```python
from build123d import *

# Parameters (mm, degrees)
EXTRUDE_1_DEPTH = 750


with BuildPart() as part:
    # Эскиз1 → Бобышка-Вытянуть1 (new body)
    with BuildSketch(Plane.XY):
        with BuildLine():
            Line((10, 14.5), (10, 13.5))
            ThreePointArc((10, 13.5), (9.853553391, 13.146446609), (9.5, 13))
            Line((9.5, 13), (-12.5, 13))
            ThreePointArc((-12.5, 13), (-12.853553391, 12.853553391), (-13, 12.5))
            Line((-13, 12.5), (-13, -9.5))
            ThreePointArc((-13, -9.5), (-13.146446609, -9.853553391), (-13.5, -10))
            Line((-13.5, -10), (-14.5, -10))
            ThreePointArc((-14.5, -10), (-14.853553391, -9.853553391), (-15, -9.5))
            Line((-15, -9.5), (-15, 15))
            Line((-15, 15), (9.5, 15))
            ThreePointArc((9.5, 15), (9.853553391, 14.853553391), (10, 14.5))
        make_face()
    extrude(amount=EXTRUDE_1_DEPTH)


solid = part.part
```
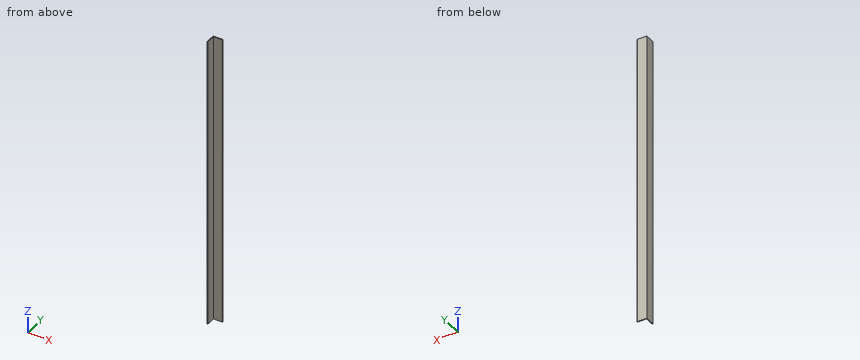
Can you work these out from the model? Positions are in its coordinate system, mm. Round coordinates to 2 decimals unless told otherwise and drop trailing zeros. Order: outer loops, then holes, each group sorted by start corner. A loop starts at its lowest first (then second) coordinate and runs counter-clockwise, first axis right, second up. Notation, with made-up numbers: (-35, -23.75) -> (6, -23.75) arc R28 cw to (6, 10.25) -> close; hole circle Ø1 at (69, 71). An arc over 180 degrees is marked (long way). Return JSON: item names as keys, results as strings. Group by question number.
1. If we section it at B-B, the plane y = -2.25: Write out the boundary of the cut face in (x, z), then the cut area to 3 significant figures.
2. If we section it at A-A, the plane z = 658.5: Write out the boundary of the cut face in (x, y).
3. If we section it at C-C, the plane x = -0.5: Write out the boundary of the cut face in (y, z), then the cut area to 3 significant figures.
4. Will this pin go through, and if not, where does the flat tip stop? pin 1 (3 mm diameter, centred on x = 7.5, z = 254, fed in from -Y).
5. I need wall thicknesses on line 1 (X direction, y = -5.5, z = 644); line 2 (Y direction, x = -0.75, z = 127). Which ranges of each line are inside material? Lowest first, please. Write a range as [from, to].
Output values:
{
 "1": {"outline": "(-15, 0) -> (-13, 0) -> (-13, 750) -> (-15, 750) -> close", "area": "1,500 mm²"},
 "2": {"outline": "(-15, -9.5) arc R0.5 ccw to (-14.5, -10) -> (-13.5, -10) arc R0.5 ccw to (-13, -9.5) -> (-13, 12.5) arc R0.5 cw to (-12.5, 13) -> (9.5, 13) arc R0.5 ccw to (10, 13.5) -> (10, 14.5) arc R0.5 ccw to (9.5, 15) -> (-15, 15) -> close"},
 "3": {"outline": "(13, 0) -> (15, 0) -> (15, 750) -> (13, 750) -> close", "area": "1,500 mm²"},
 "4": {"pin 1": "y = 13"},
 "5": {"line 1": "[-15, -13]", "line 2": "[13, 15]"}
}
